For this review, take the finished solid that the model builds, in its own axes (mm). Face numbers are marked on the shaded views. Give positions to 0.01 mm unless a question says otherwise; leave off trailing zeros. Loops run counter-clockwise (first coordinate to the right, second up) from the corner with the lowest first, then second, coordinate; pieces in that order, holes last. Notation, with made-up numbers: M 29.5,79 L 37.5,79 A6 ccw 37.5,84 Z; hole C 56.5,12.5 d8. An arc over 180 degrees is marked long. Use CSV: the item, a comma, the result in double quotes. Start each with the question number.
1. The part is to be moulded in two halves that separate along X. For the marked faces 1, 2 and 3, say which applies: pulls with the +X half, pulls with the -X half, needs draft (parallel to the pull), parting line crosses it, or undercut.
2. Take a section at B-B, the plane z = 0. Write out the cut boundary in (x, y), and give its area (3 significant figures).
3. To check wall thickness, follow line 1 (Y direction, x = -7.5, z = 0); line 2 (X direction, y = 5.3, z = 0); line 3 (Z direction, x = -5.5, y = 3). State the ranges of each line that lie inside material, in increasing order. Write a range as [from, to].
4. Take a section at A-A, the plane y = 3. Write out the cut boundary in (x, z), and give its area (3 significant figures).
5. Take a section at D-D, the plane y = 1.75. Write out the cut boundary in (x, z), and give its area (3 significant figures).
6. Take a section at C-C, the plane x = 0. Write out the cut boundary in (y, z).
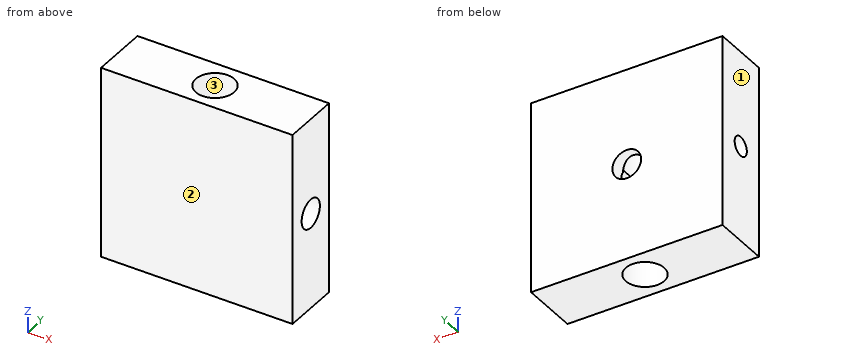
from build123d import *

# Parameters (mm, degrees)
SKETCH1_W           = 20
SKETCH1_H           = 20
BOSS_EXTRUDE1_DEPTH = 6
SKETCH2_R           = 2
CUT_EXTRUDE1_DEPTH  = 20
SKETCH3_R           = 1.5
CUT_EXTRUDE2_DEPTH  = 3
SKETCH4_R           = 1.5
CUT_EXTRUDE3_DEPTH  = 9
SKETCH5_R           = 1
CUT_EXTRUDE4_DEPTH  = 9


with BuildPart() as part:
    # Sketch1 → Boss-Extrude1 (new body)
    with BuildSketch(Plane(origin=(0, 0, 0), x_dir=(1, 0, 0), z_dir=(0, 1, 0))):
        Rectangle(SKETCH1_W, SKETCH1_H)
    extrude(amount=BOSS_EXTRUDE1_DEPTH)

    # Sketch2 → Cut-Extrude1 (cut)
    with BuildSketch(Plane.XY.offset(10)):
        with Locations((0, 3)):
            Circle(SKETCH2_R)
    extrude(amount=-CUT_EXTRUDE1_DEPTH, mode=Mode.SUBTRACT)

    # Sketch3 → Cut-Extrude2 (cut)
    with BuildSketch(Plane(origin=(0, 6, 0), x_dir=(1, 0, 0), z_dir=(0, 1, 0))):
        with Locations(Location((0, 0, 0), (0, 0, 270))):
            Circle(SKETCH3_R)
    extrude(amount=-CUT_EXTRUDE2_DEPTH, mode=Mode.SUBTRACT)

    # Sketch4 → Cut-Extrude3 (cut)
    with BuildSketch(Plane(origin=(10, 0, 0), x_dir=(0, 0, -1), z_dir=(1, 0, 0))):
        with Locations((0, 3)):
            Circle(SKETCH4_R)
    extrude(amount=-CUT_EXTRUDE3_DEPTH, mode=Mode.SUBTRACT)

    # Sketch5 → Cut-Extrude4 (cut)
    with BuildSketch(Plane.ZY.offset(10)):
        with Locations((0, 3)):
            Circle(SKETCH5_R)
    extrude(amount=-CUT_EXTRUDE4_DEPTH, mode=Mode.SUBTRACT)


solid = part.part
Result set:
1,face 1,"pulls with the -X half"
1,face 2,"needs draft"
1,face 3,"undercut"
2,outline,"M -10,0 L 10,0 L 10,1.5 L 1.32,1.5 A2 cw -1.73,2 L -10,2 Z; M -10,4 L -1.73,4 A2 cw -1.5,4.32 L -1.5,6 L -10,6 Z; M 1.5,4.5 L 10,4.5 L 10,6 L 1.5,6 Z"
2,area,"63.0 mm2"
3,line 1,"[0, 2], [4, 6]"
3,line 2,"[-10, -1.5], [1.5, 10]"
3,line 3,"[-10, -1], [1, 10]"
4,outline,"M -10,-10 L -2,-10 L -2,-1 L -10,-1 Z; M -10,1 L -2,1 L -2,10 L -10,10 Z; M 2,-10 L 10,-10 L 10,-1.5 L 2,-1.5 Z; M 2,1.5 L 10,1.5 L 10,10 L 2,10 Z"
4,area,"280 mm2"
5,outline,"M -10,-10 L -1.56,-10 L -1.56,10 L -10,10 Z; M 1.56,-10 L 10,-10 L 10,-0.83 L 1.56,-0.83 Z; M 1.56,0.83 L 10,0.83 L 10,10 L 1.56,10 Z"
5,area,"324 mm2"
6,outline,"M 0,-10 L 1,-10 L 1,10 L 0,10 Z; M 5,-10 L 6,-10 L 6,-1.5 L 5,-1.5 Z; M 5,1.5 L 6,1.5 L 6,10 L 5,10 Z"
